from build123d import *

# Parameters (mm, degrees)
F0_R     = 9.525
F1_DEPTH = 25.4
F3_DEPTH = 25.401
F4_DEPTH = 9.525
F6_DEPTH = 9.525
F7_R     = 3.81
F8_DEPTH = 12.7


with BuildPart() as f1:
    # F0 (on Front) → F1 (new body)
    with BuildSketch(Plane.XZ):
        Circle(F0_R)
    extrude(amount=-F1_DEPTH)

    # F2 (on face) → F3 (cut, through all)
    with BuildSketch(Plane.XZ):
        with BuildLine():
            ThreePointArc((4.7625, 0), (3.367596, 3.367596), (0, 4.7625))
            ThreePointArc((0, 4.7625), (-3.367596, 3.367596), (-4.7625, 0))
            ThreePointArc((-4.7625, 0), (-3.367596, -3.367596), (0, -4.7625))
            ThreePointArc((0, -4.7625), (3.367596, -3.367596), (4.7625, 0))
        make_face()
    extrude(amount=-F3_DEPTH, mode=Mode.SUBTRACT)

    # F2 (on face) → F4 (cut)
    with BuildSketch(Plane.XZ):
        with BuildLine():
            Line((4.7625, 0), (4.7625, 4.7625))
            Line((4.7625, 4.7625), (0, 4.7625))
            ThreePointArc((0, 4.7625), (3.367596, 3.367596), (4.7625, 0))
        make_face()
        with BuildLine():
            ThreePointArc((-4.7625, 0), (-3.367596, 3.367596), (0, 4.7625))
            Line((0, 4.7625), (-4.7625, 4.7625))
            Line((-4.7625, 4.7625), (-4.7625, 0))
        make_face()
        with BuildLine():
            Line((4.7625, -4.7625), (4.7625, 0))
            ThreePointArc((4.7625, 0), (3.367596, -3.367596), (0, -4.7625))
            Line((0, -4.7625), (4.7625, -4.7625))
        make_face()
        with BuildLine():
            ThreePointArc((0, -4.7625), (-3.367596, -3.367596), (-4.7625, 0))
            Line((-4.7625, 0), (-4.7625, -4.7625))
            Line((-4.7625, -4.7625), (0, -4.7625))
        make_face()
    extrude(amount=-F4_DEPTH, mode=Mode.SUBTRACT)

    # F5 (on face) → F6 (cut)
    with BuildSketch(Plane(origin=(0, 25.4, 0), x_dir=(-1, 0, 0), z_dir=(0, 1, 0))):
        Polygon((-6.324151, 3.65125), (-6.324151, -3.65125), (0, -7.3025), (6.324151, -3.65125), (6.324151, 3.65125), (0, 7.3025), align=None)
    extrude(amount=-F6_DEPTH, mode=Mode.SUBTRACT)

    # F7 (on Right) → F8 (cut, symmetric)
    with BuildSketch(Plane.YZ):
        with Locations((10.16, 0)):
            Circle(F7_R)
    extrude(amount=F8_DEPTH, both=True, mode=Mode.SUBTRACT)


solid = f1.part
Design review of the part built by this model. Coordinates are the model's own, in mm. A direction names the side the tool comes from. Coordinates: 2 decimals unless noted, no trailing zeros. Loops run counter-clockwise (first coordinate to the right, second up) from the corner with the lowest first, then second, coordinate; pieces in that order, holes last. Notation, with made-up numbers: (39.25, 83.25) -> (48.25, 83.25) arc R26 cw to (48.25, 111.25) -> close; hole circle Ø2 at (51.25, 71.25). An arc over 180 degrees is marked (long way). Use a Markdown table: item, result. Add a question column.
Item 1: We need section B-B, the plane x = 3.5. Write out the cut boundary in (y, z) (1 decimal), and give its area (3 significant figures).
Item 2: Clearance check with flat-ended pins moving along their axes: P1, Ø2, axis at x = 1.5, y = 10.5, coming from the -Z side; P2, Ø3, axis at x = -3, z = -3, coming from the +Y side (3 decimals); P3, Ø2, axis at y = 19.5, z = -1.5, coming from the -X side. State where each tip first meets the part, or that it passes through.
Item 3: We need section D-D, the plane z = -0.5. Write out the cut boundary in (x, y) (1 decimal).
Item 4: Wall thickness on L1, parallel to Y at x = 7.5, z = 0; L2, parallel to Y at x = 5.75, z = 0 (3 decimals); L3, parallel to Z at x = 6, y = 8: over which ranges is each line inside the solid? List them lowest first. Write a range as from..to.
Item 5: Machinability: for faces 1 (the flat face through (-3, 9.525, -4)), 2 (the flat face through (3.12, 20.7, 5.5)), 3 (the cylindrical face through (-6.89, 12.21, 3.21)), which of the approach directions +Z, -Z, +X, -X, +Y, -Y give a long, thin tool a straight path to every point of the face, cutting with its end or side? Answer none if there is none.
Item 6: The part is to be moulded in two halves that separate along Z. For faces 4 (the flat face through (-3.21, 20.7, 5.45)), 5 (the cylindrical face through (4.4, 12.52, -8.45)), 6 (the flat face through (0, 0, -6)), say which applies: +Z half, -Z half, draft (parallel to the pull), parting line (faces both ways), or undercut.
Numbers:
| question | item | result |
|---|---|---|
| 1 | outline | (0, -8.9) -> (25.4, -8.9) -> (25.4, -5.3) -> (15.9, -5.3) -> (15.9, -3.2) -> (12.2, -3.2) arc R3.8 cw to (9.5, -3.8) -> (9.5, -4.8) -> (0, -4.8) -> close; (0, 4.8) -> (9.5, 4.8) -> (9.5, 3.8) arc R3.8 cw to (12.2, 3.2) -> (15.9, 3.2) -> (15.9, 5.3) -> (25.4, 5.3) -> (25.4, 8.9) -> (0, 8.9) -> close |
| 1 | area | 215 mm^2 |
| 2 | P1 | stops at z = -9.51 |
| 2 | P2 | stops at y = 15.875 |
| 2 | P3 | stops at x = -9.51 |
| 3 | outline | (-9.5, 0) -> (-4.8, 0) -> (-4.8, 6.4) -> (-9.5, 6.4) -> close; (-9.5, 13.9) -> (-4.7, 13.9) -> (-4.7, 15.9) -> (-6.3, 15.9) -> (-6.3, 25.4) -> (-9.5, 25.4) -> close; (4.7, 13.9) -> (9.5, 13.9) -> (9.5, 25.4) -> (6.3, 25.4) -> (6.3, 15.9) -> (4.7, 15.9) -> close; (4.8, 0) -> (9.5, 0) -> (9.5, 6.4) -> (4.8, 6.4) -> close |
| 4 | L1 | y = 0..6.35, 13.97..25.4 |
| 4 | L2 | y = 0..6.35, 13.97..15.875 |
| 4 | L3 | z = -7.4..-3.14, 3.14..7.4 |
| 5 | face 1 | -Y |
| 5 | face 2 | +Y |
| 5 | face 3 | +X, -X |
| 6 | face 4 | undercut |
| 6 | face 5 | parting line |
| 6 | face 6 | draft |
